```python
from build123d import *

# Parameters (mm, degrees)
F0_W      = 28
F0_H      = 48
F1_DEPTH  = 25
F2_W      = 20
F2_H      = 37
F3_DEPTH  = 16
F4_R      = 3
F4_R_2    = 1.575
F5_DEPTH  = 2
F6_R      = 5
F6_R_2    = 3
F7_DEPTH  = 4
F9_DEPTH  = 9.001
F10_R     = 4.25
F11_DEPTH = 3
F13_DEPTH = 1
F17_DEPTH = 1
F18_R     = 1.74999


# Not quite as in the source:
# - a fillet or chamfer is up to 0.001 mm smaller than in the source, because OpenCascade refuses the exact size


with BuildPart() as f1:
    # F0 (on Top) → F1 (new body)
    with BuildSketch(Plane.XY):
        with Locations((-14, 24)):
            Rectangle(F0_W, F0_H)
    extrude(amount=F1_DEPTH)

    # F2 (on face) → F3 (cut)
    with BuildSketch(Plane.XY.offset(25)):
        with Locations((-14, 24)):
            Rectangle(F2_W, F2_H)
    extrude(amount=-F3_DEPTH, mode=Mode.SUBTRACT)

    # F4 (on face) → F5 (join)
    with BuildSketch(Plane.XY.offset(9)):
        with Locations((-11, 24)):
            Circle(F4_R)
        with Locations((-11, 24)):
            Circle(F4_R_2, mode=Mode.SUBTRACT)
    extrude(amount=F5_DEPTH)

    # F6 (on face) → F7 (cut)
    with BuildSketch(Plane.XY.offset(9)):
        with Locations((-11, 24)):
            Circle(F6_R)
        with Locations((-11, 24)):
            Circle(F6_R_2, mode=Mode.SUBTRACT)
    extrude(amount=-F7_DEPTH, mode=Mode.SUBTRACT)

    # F9 (cut, through all): a face of the model
    f9_faces = [f1.faces().sort_by_distance(p)[0] for p in [
        (-11, 24, 9),
    ]]
    extrude(f9_faces, amount=-F9_DEPTH, mode=Mode.SUBTRACT)

    # F10 (on face) → F11 (cut)
    with BuildSketch(Plane.XZ.offset(-42.5)):
        with Locations((-18, 15)):
            Circle(F10_R)
    extrude(amount=-F11_DEPTH, mode=Mode.SUBTRACT)

    # F12 (on face) → F13 (cut)
    with BuildSketch(Plane(origin=(0, 48, 0), x_dir=(-1, 0, 0), z_dir=(0, 1, 0))):
        with BuildLine():
            ThreePointArc((11, 20), (10.2928932188, 19.7071067812), (10, 19))
            Line((10, 19), (10, 7))
            ThreePointArc((10, 7), (10.2928932188, 6.2928932188), (11, 6))
            Line((11, 6), (17, 6))
            ThreePointArc((17, 6), (17.7071067812, 6.2928932188), (18, 7))
            ThreePointArc((18, 7), (17.7071067812, 7.7071067812), (17, 8))
            Line((17, 8), (12.5, 8))
            ThreePointArc((12.5, 8), (12.1464466094, 8.1464466094), (12, 8.5))
            Line((12, 8.5), (12, 19))
            ThreePointArc((12, 19), (11.7071067812, 19.7071067812), (11, 20))
        make_face()
    extrude(amount=-F13_DEPTH, mode=Mode.SUBTRACT)

    # F15 (on face) → F17 (cut)
    with BuildSketch(Plane.XZ.offset(-42.5)):
        Polygon((-9, 14.0925227119), (-4.75, 16.5462613559), (-4.75, 21.4537386441), (-9, 23.9074772881), (-13.25, 21.4537386441), (-13.25, 16.5462613559), align=None)
        Polygon((-9, 14.9585481157), (-12.5, 16.9792740578), (-12.5, 21.0207259422), (-9, 23.0414518843), (-5.5, 21.0207259422), (-5.5, 16.9792740578), align=None, mode=Mode.SUBTRACT)
        with BuildLine():
            Line((-10.4970194787, 17.2914120527), (-11.3840303118, 17.7531606659))
            ThreePointArc((-11.3840303118, 17.7531606659), (-11.1713992019, 17.0787809427), (-10.4970194787, 17.2914120527))
        make_face()
        with BuildLine():
            ThreePointArc((-9.4435054166, 21.0191256934), (-9.5, 21.25), (-9.4435054166, 21.4808743066))
            Line((-9.4435054166, 21.4808743066), (-11.3840303118, 17.7531606659))
            Line((-11.3840303118, 17.7531606659), (-10.4970194787, 17.2914120527))
            Line((-10.4970194787, 17.2914120527), (-9, 20.1671597149))
            Line((-9, 20.1671597149), (-9.4435054166, 21.0191256934))
        make_face()
        with BuildLine():
            ThreePointArc((-8.5564945834, 21.0191256934), (-8.5143289651, 21.1311570538), (-8.5, 21.25))
            ThreePointArc((-8.5, 21.25), (-8.5143289651, 21.3688429462), (-8.5564945834, 21.4808743066))
            ThreePointArc((-8.5564945834, 21.4808743066), (-9, 21.75), (-9.4435054166, 21.4808743066))
            ThreePointArc((-9.4435054166, 21.4808743066), (-9.5, 21.25), (-9.4435054166, 21.0191256934))
            ThreePointArc((-9.4435054166, 21.0191256934), (-9, 20.75), (-8.5564945834, 21.0191256934))
        make_face()
        with BuildLine():
            Line((-9, 20.1671597149), (-8.5564945834, 21.0191256934))
            ThreePointArc((-8.5564945834, 21.0191256934), (-9, 20.75), (-9.4435054166, 21.0191256934))
            Line((-9.4435054166, 21.0191256934), (-9, 20.1671597149))
        make_face()
        with BuildLine():
            ThreePointArc((-8.5564945834, 21.4808743066), (-8.5143289651, 21.3688429462), (-8.5, 21.25))
            ThreePointArc((-8.5, 21.25), (-8.5143289651, 21.1311570538), (-8.5564945834, 21.0191256934))
            Line((-8.5564945834, 21.0191256934), (-9, 20.1671597149))
            Line((-9, 20.1671597149), (-7.5029805213, 17.2914120527))
            Line((-7.5029805213, 17.2914120527), (-6.6159696882, 17.7531606659))
            Line((-6.6159696882, 17.7531606659), (-8.5564945834, 21.4808743066))
        make_face()
        with BuildLine():
            ThreePointArc((-7.5029805213, 17.2914120527), (-6.8286007981, 17.0787809427), (-6.6159696882, 17.7531606659))
            Line((-6.6159696882, 17.7531606659), (-7.5029805213, 17.2914120527))
        make_face()
    extrude(amount=-F17_DEPTH, mode=Mode.SUBTRACT)

    # F18 (radius 1.75 in the source; OpenCascade refuses exactly that, so slightly less here)
    f18_edges = [f1.edges().sort_by_distance(p)[0] for p in [
        (-24, 24, 9),
        (-14, 42.5, 9),
        (-4, 24, 9),
        (-14, 5.5, 9),
    ]]
    fillet(f18_edges, radius=F18_R)


solid = f1.part
```
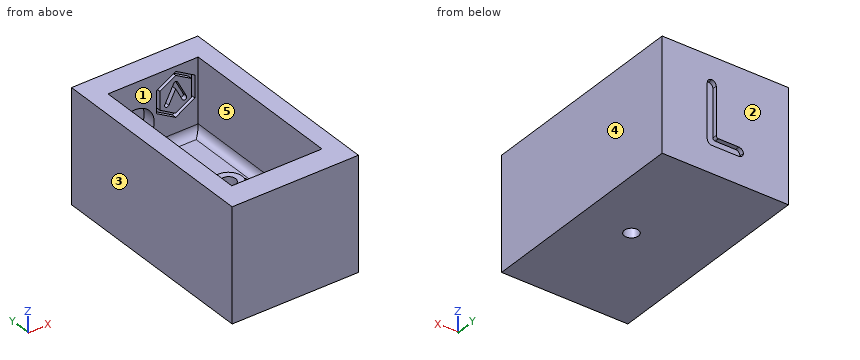
Input: part model. Units: mm. Frame: model coordinates. Face numbers are marked on the shaded views. A direction names the side the tool comes from. Coordinates: 2 decimals unless noted, no trailing zeros. Order: outer loops, then holes, each group sorted by start corner. A loop starts at its lowest first (then second) coordinate and runs counter-clockwise, first axis right, second up. Notation, with made-up numbers: (43.5, 58) - (90.5, 58) arc R24 cw to (90.5, 89) - close; hole circle Ø4 at (89.5, 37). An arc over 180 degrees is marked (long way). Put each result on its own line as item: value.
1. Contact query for flat-ended pins moving along their axis: pin 1 Ø4 at (x, y) = (-11, 24) entering from +Z; pin 2 Ø5 at (x, y) = (-10.5, 30.5) entering from +Z. Output: stop coordinate, or through.
Report:
pin 1: stops at z = 11
pin 2: stops at z = 9
2. Cut plane C-C on y = 12. Return the cut outline in (x, z), then the cut area to 3 significant figures.
Report:
outline: (-28, 0) - (0, 0) - (0, 25) - (-4, 25) - (-4, 10.75) arc R1.75 cw to (-5.75, 9) - (-22.25, 9) arc R1.75 cw to (-24, 10.75) - (-24, 25) - (-28, 25) - close
area: 381 mm2
3. Cut plane A-A on y = 24. Return the cut outline in (x, z) (3 decimals), then the cut area to 3 significant figures.
Report:
outline: (-28, 0) - (-12.575, 0) - (-12.575, 11) - (-14, 11) - (-14, 5) - (-16, 5) - (-16, 9) - (-22.25, 9) arc R1.75 cw to (-24, 10.75) - (-24, 25) - (-28, 25) - close; (-9.425, 0) - (0, 0) - (0, 25) - (-4, 25) - (-4, 10.75) arc R1.75 cw to (-5.75, 9) - (-6, 9) - (-6, 5) - (-8, 5) - (-8, 11) - (-9.425, 11) - close
area: 343 mm2
4. Draft query along Y for the marked faces 1, 2 and 3. Return one class per face: pulls with the +Y half, pulls with the -Y half, needs draft (parallel to the pull), parting line crosses it, or undercut.
Report:
face 1: undercut
face 2: pulls with the +Y half
face 3: needs draft
5. Reachability of the marked faces 4 and 5 from +Z, -Z, +X, -X, +Y, -Y: full face, straight path, thin tool, end or side. Return the list, or none.
Report:
face 4: +Z, -Z, +X, +Y, -Y
face 5: +Z
6. Line query: line 1 along Y through (x, z) = (-7.25, 11); line 2 along Y through (x, z) = (-11, 6.55) (3 decimals); line 3 along X through (y, z) = (39, 19). Output: solid intervals per line, ascending.
Report:
line 1: y = 0 to 5.5, 42.5 to 48
line 2: y = 0 to 19, 21 to 22.425, 25.575 to 27, 29 to 47
line 3: x = -28 to -24, -4 to 0
7. Cut plane B-B on z = 13.5. Return the cut outline in (x, y), then the cut area to 3 significant figures.
Report:
outline: (-28, 0) - (0, 0) - (0, 48) - (-10, 48) - (-10, 47) - (-12, 47) - (-12, 48) - (-28, 48) - close; hole (-24, 5.5) - (-4, 5.5) - (-4, 42.5) - (-14.02, 42.5) - (-14.02, 45.5) - (-21.98, 45.5) - (-21.98, 42.5) - (-24, 42.5) - close
area: 578 mm2
8. Cut plane D-D on x = -20.5. Return the cut outline in (y, z).
Report:
outline: (0, 0) - (48, 0) - (48, 25) - (42.5, 25) - (42.5, 18.44) - (45.5, 18.44) - (45.5, 11.56) - (42.5, 11.56) - (42.5, 10.75) arc R1.75 cw to (40.75, 9) - (7.25, 9) arc R1.75 cw to (5.5, 10.75) - (5.5, 25) - (0, 25) - close
